Part model, mm, in its own coordinate system. Face numbers are marked on the shaded views. A direction names the side the tool comes from. Give positions to 0.01 mm unless a question says otherwise; leave off trailing zeros. Order: outer loops, then holes, each group sorted by start corner. A loop starts at its lowest first (then second) coordinate and runs counter-clockwise, first axis right, second up.
from build123d import *

# Parameters (mm, degrees)
SKETCH1_W           = 152.4
SKETCH1_H           = 228.6
BOSS_EXTRUDE1_DEPTH = 127
CUT_EXTRUDE1_DEPTH  = 153.4
CUT_EXTRUDE2_DEPTH  = 153.4
SHELL1_T            = -2


with BuildPart() as part:
    # Sketch1 → Boss-Extrude1 (new body)
    with BuildSketch(Plane(origin=(0, 0, 0), x_dir=(1, 0, 0), z_dir=(0, 1, 0))):
        Rectangle(SKETCH1_W, SKETCH1_H)
    extrude(amount=BOSS_EXTRUDE1_DEPTH)

    # Sketch2 → Cut-Extrude1 (cut, through all)
    with BuildSketch(Plane(origin=(76.2, 0, 0), x_dir=(0, 0, -1), z_dir=(1, 0, 0))):
        Polygon((-101.6, 127), (-114.3, 25.4), (-114.3, 127), align=None)
        Polygon((-114.3, 6.35), (-114.3, 0), (-104.775, 0), align=None)
    extrude(amount=-CUT_EXTRUDE1_DEPTH, mode=Mode.SUBTRACT)

    # Sketch3 → Cut-Extrude2 (cut, through all)
    with BuildSketch(Plane(origin=(76.2, 0, 0), x_dir=(0, 0, -1), z_dir=(1, 0, 0))):
        Polygon((107.3, 7.216451884), (107.3, 116), (107.3, 124), (112.3, 124), (112.3, 116), (114.3, 116), (114.3, 3.175), align=None)
    extrude(amount=-CUT_EXTRUDE2_DEPTH, mode=Mode.SUBTRACT)

    # Shell1
    shell1_openings = [part.faces().sort_by_distance(p)[0] for p in [
        (0, 127, -6.35),
        (0, 76.2, 107.95),
    ]]
    offset(amount=SHELL1_T, openings=shell1_openings, kind=Kind.INTERSECTION)


solid = part.part
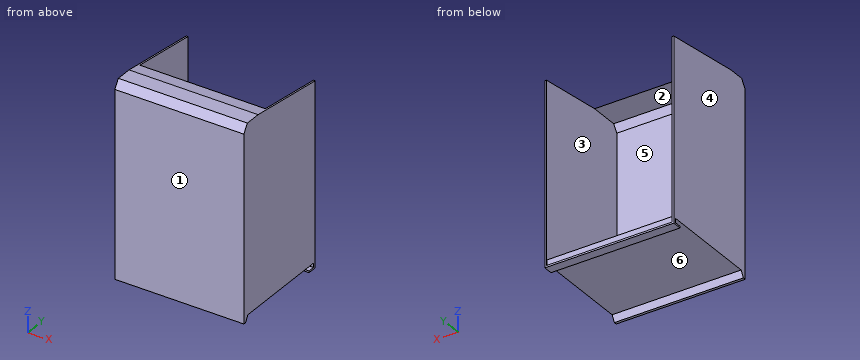
Item 1: Drop flat-ended pins along their axis: P1, Ø1, axis at x = -19, z = -113, coming from the -Y side; P2, Ø10, axis at x = 26.5, z = -59.5, coming from the +Y side; P3, Ø3.5, axis at x = 33.5, z = -107.5, coming from the +Y side; P4, Ø3, axis at x = 2.5, y = 58.5, coming from the -Z side. Give the stop position or say it passes through.
Item 2: Which spindle directions (+Z, -Z, +X, -X, +Y, -Y) get a long thin tool onto all of the face, cutting with end or side? Do the marked faces 1 and 2. Say none if no direction does.
Item 3: Band-saw the part on B-B on x = 5.5. List the corners of the cut face in (y, z) (3 decimals), plus the area to 3 significant figures.
Item 4: Band-saw the part on C-C on z = 17. List the corners of the cut face in (x, y), plus the area to 3 significant figures.
Item 5: Band-saw the part on D-D on y = 47. List the corners of the cut face in (x, z), plus the area to 3 significant figures.
Item 6: Pull direction X, two halves, no side cores. Call the marked faces 3, 4, 5 and 6: released by +X, released by -X, zero draft, split by the parting line, or undercut.
Item 7: Band-saw the part on A-A on y = 16.5. List the corners of the cut face in (x, z), plus the area to 3 significant figures.
Item 8: Drill centre lines: probe 1 along X at (y, z) = (16.5, -45.5); probe 2 along Z at (x, y) = (50.5, 117.5); probe 3 along Y at (x, z) = (24, -29.5). Where is each one in solid material? Low to high.
Working result:
1. P1: stops at y = 0
1. P2: stops at y = 2
1. P3: stops at y = 126
1. P4: stops at z = -107.3
2. face 1: +Z, -Z, +X, -X, -Y
2. face 2: +Y
3. outline: (0, -114.3) - (3.175, -114.3) - (7.216, -107.3) - (124, -107.3) - (124, -112.3) - (116, -112.3) - (116, -114.3) - (127, -114.3) - (127, -112.3) - (126, -112.3) - (126, -105.3) - (6.062, -105.3) - (2.02, -112.3) - (2, -112.3) - (2, 104.169) - (7.42, 112.3) - (41.4, 112.3) - (25.4, 114.3) - (6.35, 114.3) - (0, 104.775) - close
3. area: 800 mm2
4. outline: (-76.2, 0) - (76.2, 0) - (76.2, 127) - (74.2, 127) - (74.2, 2) - (-74.2, 2) - (-74.2, 127) - (-76.2, 127) - close
4. area: 805 mm2
5. outline: (-76.2, -107.3) - (76.2, -107.3) - (76.2, 111.6) - (74.2, 111.6) - (74.2, -105.3) - (-74.2, -105.3) - (-74.2, 111.6) - (-76.2, 111.6) - close
5. area: 1,170 mm2
6. face 3: undercut
6. face 4: released by -X
6. face 5: undercut
6. face 6: zero draft
7. outline: (-76.2, -107.3) - (76.2, -107.3) - (76.2, 114.3) - (-76.2, 114.3) - close; hole (-74.2, -105.3) - (74.2, -105.3) - (74.2, 112.3) - (-74.2, 112.3) - close
7. area: 1,480 mm2
8. probe 1: x = -76.2 to -74.2, 74.2 to 76.2
8. probe 2: z = -114.3 to -112.3, -107.3 to -105.3
8. probe 3: y = 0 to 2
